Geometry check sheet. Reference: the model listing, model coordinates, mm. A direction names the side the tool comes from. Give positions to 0.01 mm unless a question says otherwise; leave off trailing zeros. Loops run counter-clockwise (first coordinate to the right, second up) from the corner with the lowest first, then second, coordinate; pieces in that order, holes last. Notation, with made-up numbers: (68.5, 76) -> (98.5, 76) arc R23 ccw to (98.5, 96) -> close; hole circle Ø9 at (6, -38). An arc over 180 degrees is marked (long way). Write item = value, one per line.
```python
from build123d import *

# Parameters (mm, degrees)
F0_W      = 80.2132
F0_H      = 55.1688
F1_DEPTH  = 25
F3_W      = 80.0983905792
F3_H      = 66.7644366622
F4_DEPTH  = 14.8
F6_W      = 67.9705310613
F6_H      = 14.8716745898
F7_DEPTH  = 99
F8_R      = 5
F9_W      = 35.595134832
F9_H      = 10.9548680484
F10_DEPTH = 10
F11_R     = 7
F12_R     = 2
F13_R     = 10


# Not quite as in the source:
# - a pattern or mirror of a feature is missing from the dataset's text; its kind, count and spacing are read off the source's solid


with BuildPart() as f1:
    # F0 (on Top) → F1 (new body)
    with BuildSketch(Plane.XY):
        with Locations((40.1066, 27.5844)):
            Rectangle(F0_W, F0_H)
    extrude(amount=F1_DEPTH)

    # F3 (on offset) → F4 (join)
    with BuildSketch(Plane.XZ.offset(-55)):
        with Locations((40.0491952896, 33.3822183311)):
            Rectangle(F3_W, F3_H)
    extrude(amount=F4_DEPTH)

    # F6 (on Front) → F7 (cut)
    with BuildSketch(Plane.XZ):
        with Locations((40.3414806351, 7.4358372949)):
            Rectangle(F6_W, F6_H)
    extrude(amount=-F7_DEPTH, mode=Mode.SUBTRACT)

    # F8
    f8_edges = [f1.edges().sort_by_distance(p)[0] for p in [
        (40.1066, 0, 25),
    ]]
    fillet(f8_edges, radius=F8_R)

    # F9 (on Right) → F10 (join)
    with BuildSketch(Plane.YZ):
        with Locations((22.8417287581, 30.5123161525)):
            Rectangle(F9_W, F9_H)
    f10 = extrude(amount=F10_DEPTH)

    # F10_copies: F10 across plane
    add(f10.mirror(Plane(origin=(40, 0, 0), x_dir=(0, 0, 1), z_dir=(1, 0, 0))))

    # F11
    f11_edges = [f1.edges().sort_by_distance(p)[0] for p in [
        (10, 22.622081, 35.98975),
        (70, 22.622081, 35.98975),
    ]]
    fillet(f11_edges, radius=F11_R)

    # F12
    f12_edges = [f1.edges().sort_by_distance(p)[0] for p in [
        (0, 22.622081, 35.98975),
        (80, 22.622081, 35.98975),
    ]]
    fillet(f12_edges, radius=F12_R)

    # F13
    f13_edges = [f1.edges().sort_by_distance(p)[0] for p in [
        (40.049195, 40.2, 66.764437),
    ]]
    fillet(f13_edges, radius=F13_R)


solid = f1.part
```
Item 1: Section check D-D, the plane z = 52. Record the cut outline in (x, y).
Answer:
outline = (0, 40.2) -> (80.1, 40.2) -> (80.1, 55) -> (0, 55) -> close
Item 2: Gauge pin test, flat ends, axial feed: pin 1 (12 mm diameter, centred on x = 61, y = 30, fed in from -Z); pin 2 (9.5 mm diameter, centred on x = 43.5, z = 47, fed in from -Y); pin 3 (0.8 mm diameter, centred on x = 77.5, y = 21, fed in from +Z). Record the tip position at first contact, or that the pin passes through.
Answer:
pin_1 = 14.87
pin_2 = 40.2
pin_3 = 35.99
Item 3: Section check B-B, the plane y = 18.5. Record the cut outline in (x, z), plus the area to 3 significant figures.
Answer:
outline = (0, 0) -> (6.36, 0) -> (6.36, 14.87) -> (74.33, 14.87) -> (74.33, 0) -> (80.21, 0) -> (80.21, 25) -> (0, 25) -> close; (0, 25.03) -> (10, 25.03) -> (10, 28.99) arc R7 ccw to (3, 35.99) -> (2, 35.99) arc R2 ccw to (0, 33.99) -> close; (70, 25.03) -> (80, 25.03) -> (80, 33.99) arc R2 ccw to (78, 35.99) -> (77, 35.99) arc R7 ccw to (70, 28.99) -> close
area = 1,190 mm^2
Item 4: Section check C-C, the plane x = 11.5. Record the cut outline in (y, z).
Answer:
outline = (0, 14.87) -> (55.17, 14.87) -> (55.17, 25) -> (55, 25) -> (55, 66.76) -> (50.2, 66.76) arc R10 ccw to (40.2, 56.76) -> (40.2, 25) -> (5, 25) arc R5 ccw to (0, 20) -> close
Item 5: Section check A-A, the plane z = 10.5. Record the cut outline in (x, y).
Answer:
outline = (0, 0) -> (6.36, 0) -> (6.36, 55.17) -> (0, 55.17) -> close; (74.33, 0) -> (80.21, 0) -> (80.21, 55.17) -> (74.33, 55.17) -> close
Item 6: Thickness scan on L1, parallel to X at y = 38, z = 27; L2, parallel to X at y = 34, z = 5; L3, parallel to Y at x = 22.5, z = 50. Record the ranges inside material, lowest first. Write a range as [from, to].
Answer:
L1 = [0, 10], [70, 80]
L2 = [0, 6.36], [74.33, 80.21]
L3 = [40.2, 55]
Item 7: Tool access check on faces 1 (the flat face through (74.327, 27, 7)), 2 (the cylindrical face through (79.4, 22.87, 35.42)), 3 (the cylindrical face through (0.6, 22.87, 35.42)), 4 (the cylindrical face through (72.1, 22.87, 33.99)), 5 (the flat face through (75, 5.044, 30)). Record the directions out of +Z, -Z, +X, -X, +Y, -Y that give a thin tool (end or side, any length) a straight path to the whole face; none if there is none.
Answer:
face_1 = -Z, +Y, -Y
face_2 = +Z, +X, -Y
face_3 = +Z, -X, -Y
face_4 = +Z, -Y
face_5 = +Z, +X, -X, -Y
